Check sheet for the modelled part. Datum: model origin and axes. Units: mm. Face numbers are marked on the shaded views. A direction names the side the tool comes from. Round coordinates to 2 decimals unless told otherwise and drop trailing zeros. Order: outer loops, then holes, each group sorted by start corner. A loop starts at its lowest first (then second) coordinate and runs counter-clockwise, first axis right, second up.
Q1. Cross-section at B-B on z = 3.5. Record the cut outline in (x, y), then the cut area to 3 significant figures.
Q2. Mould release check, pull along X, two halves, no side actions. Record for the marked faces 3, 4 and 5: +X half, -X half, draft (parallel to the pull), parting line (faces both ways), or undercut.
Q3. Set-up check for the marked faces 1 and 2: record each of +Z, -Z, +X, -X, +Y, -Y from which the full face is reachable in a straight line by a thin tool's end or side.
Q4. Depth check by flat-ended pin: P1, Ø4, axis at x = 2, y = 1.5, coming from the +Z side; P2, Ø1, axis at x = -6.5, y = 13, coming from the -Z side; P3, Ø1.5, axis at x = -4, z = 1.5, coming from the +Y side. Enter the tip coordinate at first touch or a pass-through.
Q5. Scan lines: probe 1 along X at (y, z) = (2.75, 9); probe 2 along X at (y, z) = (5, 4.5); probe 3 along Z at (x, y) = (4, 0.75). Record each from-to range of solid material in increasing order.
from build123d import *

# Parameters (mm, degrees)
F1_DEPTH = 10
F2_R     = 4.99999
F3_R     = 4.99999


# Not quite as in the source:
# - a fillet or chamfer is up to 0.001 mm smaller than in the source, because OpenCascade refuses the exact size


with BuildPart() as f1:
    # F0 (on Top) → F1 (new body)
    with BuildSketch(Plane.XY):
        with BuildLine():
            Line((-11.7916028897, 0), (-1.65, 0))
            Line((-1.65, 0), (-1.65, 2.85))
            ThreePointArc((-1.65, 2.85), (-1.2298373876, 7.5096747752), (2.75, 5.05))
            ThreePointArc((2.75, 5.05), (2.4596747752, 3.8201626124), (1.65, 2.85))
            Line((1.65, 2.85), (1.65, 0))
            Line((1.65, 0), (11.2060164511, 0))
            Line((11.2060164511, 0), (11.2060164511, 15.24))
            Line((11.2060164511, 15.24), (-11.7916028897, 15.24))
            Line((-11.7916028897, 15.24), (-11.7916028897, 0))
        make_face()
    extrude(amount=F1_DEPTH)

    # F2 (radius 5 in the source; OpenCascade refuses exactly that, so slightly less here)
    f2_edges = [f1.edges().sort_by_distance(p)[0] for p in [
        (11.206016, 7.62, 10),
        (11.206016, 7.62, 0),
        (-11.791603, 7.62, 0),
        (-11.791603, 7.62, 10),
    ]]
    fillet(f2_edges, radius=F2_R)

    # F3 (radius 5 in the source; OpenCascade refuses exactly that, so slightly less here)
    f3_edges = [f1.edges().sort_by_distance(p)[0] for p in [
        (-0.292793, 15.24, 10),
        (-10.32714, 0, 1.464463),
        (9.741553, 0, 1.464463),
    ]]
    fillet(f3_edges, radius=F3_R)


solid = f1.part
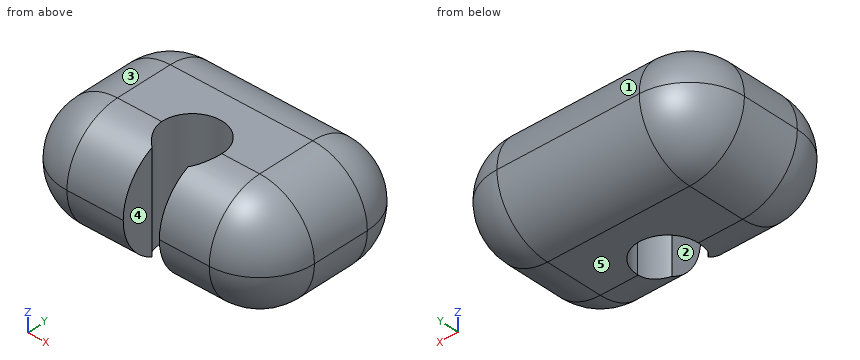
Results found:
1. outline: (-11.56, 5) arc R4.77 ccw to (-6.79, 0.23) - (-1.65, 0.23) - (-1.65, 2.85) arc R2.75 cw (long way) to (1.65, 2.85) - (1.65, 0.23) - (6.21, 0.23) arc R4.77 ccw to (10.98, 5) - (10.98, 10.24) arc R4.77 ccw to (6.21, 15.01) - (-6.79, 15.01) arc R4.77 ccw to (-11.56, 10.24) - close
1. area: 282 mm2
2. face 3: -X half
2. face 4: undercut
2. face 5: draft
3. face 1: +Z, +X, -X, +Y
3. face 2: +Z, -Z, -Y
4. P1: stops at z = 9.76
4. P2: stops at z = 0.54
4. P3: stops at y = 14.42
5. probe 1: x = -8.78 to -1.65, 1.65 to 8.19
5. probe 2: x = -11.77 to -2.75, 2.75 to 11.18
5. probe 3: z = 2.37 to 7.63
